```python
from build123d import *

# Parameters (mm, degrees)
F0_R     = 6.35
F1_DEPTH = 3.175


# Not quite as in the source:
# - a feature names something its author has since deleted; it is built from what else it names


with BuildPart() as f1:
    # F0 (on Top) → F1 (new body)
    with BuildSketch(Plane.XY):
        Polygon((-70.7512, 63.5), (-76.2, 63.5), (-76.2, -63.5), (-70.7512, -63.5), (-70.7512, -60.325), (-45.3512, -60.325), (-45.3512, -63.5), (-6.35, -63.5), (-6.35, -60.325), (31.75, -60.325), (31.75, -63.5), (70.7512, -63.5), (70.7512, -60.325), (96.1512, -60.325), (96.1512, -63.5), (101.6, -63.5), (101.6, 63.5), (96.1512, 63.5), (96.1512, 60.325), (70.7512, 60.325), (70.7512, 63.5), (31.75, 63.5), (31.75, 60.325), (-6.35, 60.325), (-6.35, 63.5), (-45.3512, 63.5), (-45.3512, 60.325), (-70.7512, 60.325), align=None)
        with Locations((-25.4, -38.1)):
            Circle(F0_R, mode=Mode.SUBTRACT)
        Polygon((-70.7512, -50.8), (-70.7512, -47.625), (-45.3512, -47.625), (-6.35, -47.625), (31.75, -47.625), (70.7512, -47.625), (96.1512, -47.625), (96.1512, -50.8), (70.7512, -50.8), (31.75, -50.8), (-6.35, -50.8), (-45.3512, -50.8), align=None, mode=Mode.SUBTRACT)
        with Locations((63.5, -38.1)):
            Circle(F0_R, mode=Mode.SUBTRACT)
        with Locations((-25.4, 38.1)):
            Circle(F0_R, mode=Mode.SUBTRACT)
        Polygon((96.1512, 50.8), (96.1512, 47.625), (70.7512, 47.625), (31.75, 47.625), (-6.35, 47.625), (-45.3512, 47.625), (-70.7512, 47.625), (-70.7512, 50.8), (-45.3512, 50.8), (-6.35, 50.8), (31.75, 50.8), (70.7512, 50.8), align=None, mode=Mode.SUBTRACT)
        with Locations((63.5, 38.1)):
            Circle(F0_R, mode=Mode.SUBTRACT)
    extrude(amount=F1_DEPTH)


solid = f1.part
```
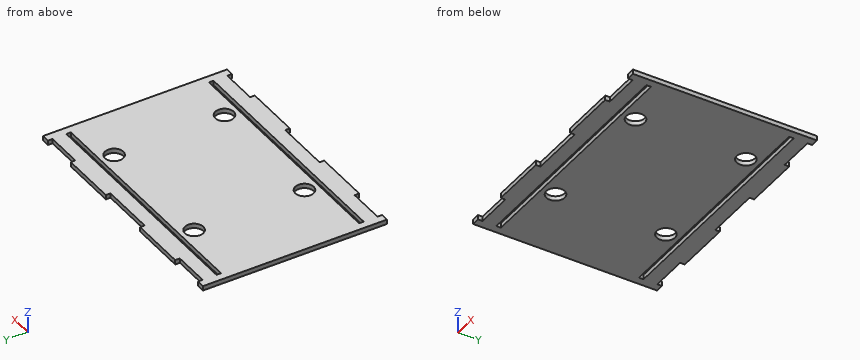
Work out the finished part from the listing and answer in its coordinate system (mm). Coordinates: 2 decimals unless noted, no trailing zeros. Write each loop counter-clockwise with the first axis right and the second up, starting at its lowest first coordinate (ties: lowest second). Pieces come first, ordered by that corner, then holes. Notation, with made-up numbers: (2, 5.25) - (27, 5.25) arc R22 ccw to (27, 31.25) - close; hole circle Ø6 at (63, 37). An arc over 180 degrees is marked (long way). Answer as a JSON object with one key per item and string values.
Q1. Find section D-D (z = 1.65). State how many separate pieces and enclosed holes the cut face has, plus the area to 3 significant figures.
Results list:
{"separate pieces": "1", "enclosed holes": "6", "area": "20,400 mm^2"}
Q2. Find section B-B (y = 38.1). Write down the section's boundary in (x, z) (3 decimals), plus the area to 3 significant figures.
Results list:
{"outline": "(-76.2, 0) - (-31.75, 0) - (-31.75, 3.175) - (-76.2, 3.175) - close; (-19.05, 0) - (57.15, 0) - (57.15, 3.175) - (-19.05, 3.175) - close; (69.85, 0) - (101.6, 0) - (101.6, 3.175) - (69.85, 3.175) - close", "area": "484 mm^2"}
Q3. Find section A-A (x = -25.4). Write down the section's boundary in (y, z) (3 decimals).
Results list:
{"outline": "(-63.5, 0) - (-50.8, 0) - (-50.8, 3.175) - (-63.5, 3.175) - close; (-47.625, 0) - (-44.45, 0) - (-44.45, 3.175) - (-47.625, 3.175) - close; (-31.75, 0) - (31.75, 0) - (31.75, 3.175) - (-31.75, 3.175) - close; (44.45, 0) - (47.625, 0) - (47.625, 3.175) - (44.45, 3.175) - close; (50.8, 0) - (63.5, 0) - (63.5, 3.175) - (50.8, 3.175) - close"}
Q4. Consider L1, parallel to Y at x = 82.5, z = 0.2 (3 decimals); L2, parallel to Y at x = 63.5, z = 1.95 (3 decimals); L3, parallel to X at y = 49, z = 3.05. Determine where each line is inside the solid, lowest interval first. Write a range as from..to.
Results list:
{"L1": "y = -60.325..-50.8, -47.625..47.625, 50.8..60.325", "L2": "y = -63.5..-50.8, -47.625..-44.45, -31.75..31.75, 44.45..47.625, 50.8..63.5", "L3": "x = -76.2..-70.75, 96.15..101.6"}
Q5. Find section C-C (x = 23). Write down the section's boundary in (y, z) (3 decimals).
Results list:
{"outline": "(-60.325, 0) - (-50.8, 0) - (-50.8, 3.175) - (-60.325, 3.175) - close; (-47.625, 0) - (47.625, 0) - (47.625, 3.175) - (-47.625, 3.175) - close; (50.8, 0) - (60.325, 0) - (60.325, 3.175) - (50.8, 3.175) - close"}
